from build123d import *

# Parameters (mm, degrees)
EXTRUDE_START       = -864.980118087
EXTRUDE_1_DEPTH     = 864.980118087
CUT_EXTRUDE_1_DEPTH = 867.94325344


# Read off the part's stored shape, not the designer's step: Бобышка-Вытянуть1
with BuildPart() as part:
    # Бобышка-Вытянуть1 outline → Бобышка-Вытянуть1 (new body)
    with BuildSketch(Plane.XY.offset(EXTRUDE_START)):
        with BuildLine():
            Line((-15, -23), (-15, -47))
            ThreePointArc((-15, -47), (-14.121320344, -49.121320344), (-12, -50))
            Line((-12, -50), (12, -50))
            ThreePointArc((12, -50), (14.121320344, -49.121320344), (15, -47))
            Line((15, -47), (15, -23))
            ThreePointArc((15, -23), (14.121320344, -20.878679656), (12, -20))
            Line((12, -20), (-12, -20))
            ThreePointArc((-12, -20), (-14.121320344, -20.878679656), (-15, -23))
        make_face()
        with BuildLine():
            ThreePointArc((-11, -48), (-12.414213562, -47.414213562), (-13, -46))
            Line((-13, -46), (-13, -24))
            ThreePointArc((-13, -24), (-12.414213562, -22.585786438), (-11, -22))
            Line((-11, -22), (11, -22))
            ThreePointArc((11, -22), (12.414213562, -22.585786438), (13, -24))
            Line((13, -24), (13, -46))
            ThreePointArc((13, -46), (12.414213562, -47.414213562), (11, -48))
            Line((11, -48), (-11, -48))
        make_face(mode=Mode.SUBTRACT)
    extrude(amount=EXTRUDE_1_DEPTH)

    # Эскиз2 → Вырез-Вытянуть1 (cut, through all)
    with BuildSketch(Plane.ZY.offset(15)):
        Polygon((-682.136609507, -20), (-674.48972614, -50), (-864.980118087, -50), (-864.980118087, -20), align=None)
    extrude(amount=-CUT_EXTRUDE_1_DEPTH, mode=Mode.SUBTRACT)


solid = part.part
Part model, mm, in its own coordinate system. A direction names the side the tool comes from. Coordinates: 2 decimals unless noted, no trailing zeros. Order: outer loops, then holes, each group sorted by start corner. A loop starts at its lowest first (then second) coordinate and runs counter-clockwise, first axis right, second up. Notation, with made-up numbers: (-31.75, 17.25) - (-26.75, 17.25) arc R33 ccw to (-26.75, 47.25) - close; hole circle Ø5 at (60, 35). An arc over 180 degrees is marked (long way). Use CSV: the item, a comma, the result in double quotes.
Item 1: Saw through at B-B on y = -28.5. Give the cut face in (x, z).
Solved:
outline,"(-15, -679.97) - (-13, -679.97) - (-13, 0) - (-15, 0) - close; (13, -679.97) - (15, -679.97) - (15, 0) - (13, 0) - close"
Item 2: Saw through at A-A on z = -487. Give the cut face in (x, y).
Solved:
outline,"(-15, -47) arc R3 ccw to (-12, -50) - (12, -50) arc R3 ccw to (15, -47) - (15, -23) arc R3 ccw to (12, -20) - (-12, -20) arc R3 ccw to (-15, -23) - close; hole (-13, -46) arc R2 ccw to (-11, -48) - (11, -48) arc R2 ccw to (13, -46) - (13, -24) arc R2 ccw to (11, -22) - (-11, -22) arc R2 ccw to (-13, -24) - close"
Item 3: Drop a flat-ended pin along its axis: P1, Ø8, axis at x = -8, y = -33, coming from the +Z side. Give the stop position or say it passes through.
Solved:
P1,"passes through"
Item 4: Probe probe 1 along Y at (x, z) = (4, -324.5); probe 2 along X at (y, z) = (-38.25, -195); probe 3 along Y at (x, z) = (-11.5, -531). List the from-to ranges inside material, lowest first.
Solved:
probe 1,"y = -50 to -48, -22 to -20"
probe 2,"x = -15 to -13, 13 to 15"
probe 3,"y = -50 to -47.94, -22.06 to -20"
Item 5: 3-axis set-ups, long thin cutter, end or side, ignore diameter. For faces 4 (the face through (0, -48, -342)), 5 (the face through (15, -35, -345)): which of +Z, -Z, +X, -X, +Y, -Y reach the whole face in a straight line?
Solved:
face 4,"+Z, -Z"
face 5,"+Z, -Z, +X, +Y, -Y"
Item 6: Mould opens along Y. For faces 1 (the face through (-13.543, -34.79, -678.367)), 2 (the face through (0, -20, -346)), 3 (the face through (0, -22, -346)) say: +Y half, -Y half, draft (parallel to the pull), parting line (faces both ways), or undercut.
Solved:
face 1,"-Y half"
face 2,"+Y half"
face 3,"undercut"
Item 7: Saw through at C-C on x = 2. Give the cut face in (y, z), and give its area (3 significant figures).
Solved:
outline,"(-50, -674.49) - (-48, -675) - (-48, 0) - (-50, 0) - close; (-22, -681.63) - (-20, -682.14) - (-20, 0) - (-22, 0) - close"
area,"2,710 mm²"
